Check sheet for the modelled part. Datum: model origin and axes. Units: mm. Coordinates: 2 decimals unless noted, no trailing zeros. Loops run counter-clockwise (first coordinate to the right, second up) from the corner with the lowest first, then second, coordinate; pieces in that order, holes last.
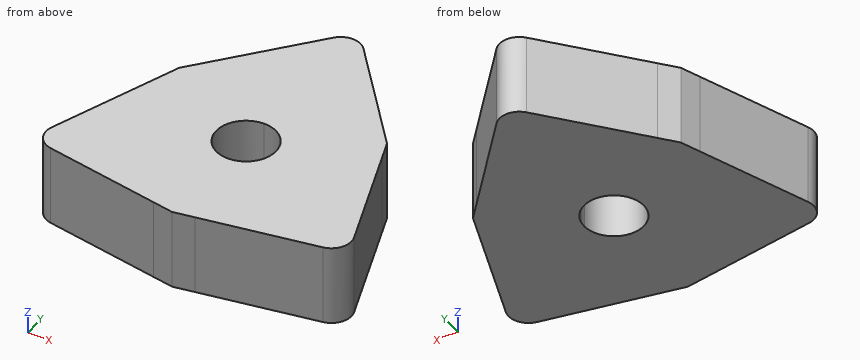
from build123d import *

# Parameters (mm, degrees)
F1_DEPTH = 3.175
F2_R     = 0.79375


with BuildPart() as f1:
    # F0 (on Top) → F1 (new body)
    with BuildSketch(Plane.XY):
        with BuildLine():
            ThreePointArc((0, 4.7625), (2.0127194988, 4.316290823), (3.648286699, 3.061275945))
            Line((3.648286699, 3.061275945), (0, 7.4091347254))
            Line((0, 7.4091347254), (0, 4.7625))
        make_face()
        with BuildLine():
            ThreePointArc((-3.6482866444, 3.0612760102), (-2.0127194603, 4.316290841), (0, 4.7625))
            Line((0, 4.7625), (0, 7.4091347254))
            Line((0, 7.4091347254), (-3.6482866444, 3.0612760102))
        make_face()
        with BuildLine():
            ThreePointArc((0.8269994491, -4.6901469232), (3.6482866613, -3.06127599), (4.7625, 0))
            ThreePointArc((4.7625, 0), (4.6901469251, 0.8269994386), (4.4752861117, 1.6288709182))
            ThreePointArc((4.4752861117, 1.6288709182), (4.1244460044, 2.3812499673), (3.648286699, 3.061275945))
            ThreePointArc((3.648286699, 3.061275945), (2.0127194988, 4.316290823), (0, 4.7625))
            ThreePointArc((0, 4.7625), (-2.0127194603, 4.316290841), (-3.6482866444, 3.0612760102))
            ThreePointArc((-3.6482866444, 3.0612760102), (-4.1244459867, 2.3812499979), (-4.4752861166, 1.6288709047))
            ThreePointArc((-4.4752861166, 1.6288709047), (-4.1244459762, -2.3812500162), (-0.8269994386, -4.6901469251))
            ThreePointArc((-0.8269994386, -4.6901469251), (5.3e-09, -4.7625), (0.8269994491, -4.6901469232))
        make_face()
        with BuildLine():
            ThreePointArc((1.18745, 0), (-0.8396539473, -0.8396539473), (0, 1.18745))
            ThreePointArc((0, 1.18745), (0.8396539473, 0.8396539473), (1.18745, 0))
        make_face(mode=Mode.SUBTRACT)
        with BuildLine():
            ThreePointArc((4.4752861117, 1.6288709182), (4.6901469251, 0.8269994386), (4.7625, 0))
            ThreePointArc((4.7625, 0), (3.6482866613, -3.06127599), (0.8269994491, -4.6901469232))
            Line((0.8269994491, -4.6901469232), (6.4164988923, -3.7045673627))
            Line((6.4164988923, -3.7045673627), (4.4752861117, 1.6288709182))
        make_face()
        with BuildLine():
            Line((-6.4164988923, -3.7045673627), (-0.8269994386, -4.6901469251))
            ThreePointArc((-0.8269994386, -4.6901469251), (-4.1244459762, -2.3812500162), (-4.4752861166, 1.6288709047))
            Line((-4.4752861166, 1.6288709047), (-6.4164988923, -3.7045673627))
        make_face()
        with BuildLine():
            ThreePointArc((3.648286699, 3.061275945), (4.1244460044, 2.3812499673), (4.4752861117, 1.6288709182))
            Line((4.4752861117, 1.6288709182), (4.188072213, 2.4179846196))
            Line((4.188072213, 2.4179846196), (3.648286699, 3.061275945))
        make_face()
        with BuildLine():
            Line((-4.188072213, 2.4179846196), (-4.4752861166, 1.6288709047))
            ThreePointArc((-4.4752861166, 1.6288709047), (-4.1244459867, 2.3812499979), (-3.6482866444, 3.0612760102))
            Line((-3.6482866444, 3.0612760102), (-4.188072213, 2.4179846196))
        make_face()
        with BuildLine():
            Line((0, -4.8359692391), (0.8269994491, -4.6901469232))
            ThreePointArc((0.8269994491, -4.6901469232), (5.3e-09, -4.7625), (-0.8269994386, -4.6901469251))
            Line((-0.8269994386, -4.6901469251), (0, -4.8359692391))
        make_face()
    extrude(amount=F1_DEPTH)

    # F2
    f2_edges = [f1.edges().sort_by_distance(p)[0] for p in [
        (0, 7.409135, 1.5875),
        (-6.416499, -3.704567, 1.5875),
        (6.416499, -3.704567, 1.5875),
    ]]
    fillet(f2_edges, radius=F2_R)


solid = f1.part
(1) Scan lines: line 1 along Y through (x, z) = (0, 2.4); line 2 along X through (y, z) = (0, 0.75); line 3 along X through (y, z) = (-0.75, 2.7). Record each from-to range of solid material in increasing order.
(2) Gauge pin test, flat ends, axial feed: P1, Ø1, axis at y = 2.5, z = 0.5, coming from the -X side; P2, Ø1.5, axis at x = 1.5, z = 1.5, coming from the +Y side. Record the tip position at first contact, or that the pin passes through.
(3) Section check A-A, the plane x = 0.25. Enter the section's corners in (y, z) (3 decimals).
(4) Section check D-D, the plane y = 5.75. Enter the section's corners in (x, z) (3 decimals).
(5) Section check C-C, the plane y = -0.5. Enter the section's corners in (x, z) (3 decimals).
(6) Section check B-B, the plane z = 2.5. Enter the section's corners in (x, y), plus the area to 3 significant figures.
Determined:
1. line 1: y = -4.84 to -1.19, 1.19 to 6.97
1. line 2: x = -5.07 to -1.19, 1.19 to 5.07
1. line 3: x = -5.34 to -0.92, 0.92 to 5.34
2. P1: stops at x = -4.34
2. P2: stops at y = 6.52
3. outline: (-4.792, 0) - (-1.161, 0) - (-1.161, 3.175) - (-4.792, 3.175) - close; (1.161, 0) - (6.928, 0) - (6.928, 3.175) - (1.161, 3.175) - close
4. outline: (-1.392, 0) - (1.392, 0) - (1.392, 3.175) - (-1.392, 3.175) - close
5. outline: (-5.25, 0) - (-1.077, 0) - (-1.077, 3.175) - (-5.25, 3.175) - close; (1.077, 0) - (5.25, 0) - (5.25, 3.175) - (1.077, 3.175) - close
6. outline: (-6.09, -2.82) arc R0.79 ccw to (-5.48, -3.87) - (0, -4.84) - (5.48, -3.87) arc R0.79 ccw to (6.09, -2.82) - (4.19, 2.42) - (0.61, 6.68) arc R0.79 ccw to (-0.61, 6.68) - (-4.19, 2.42) - close; hole circle Ø2.37 at (0, 0)
6. area: 88.1 mm2
